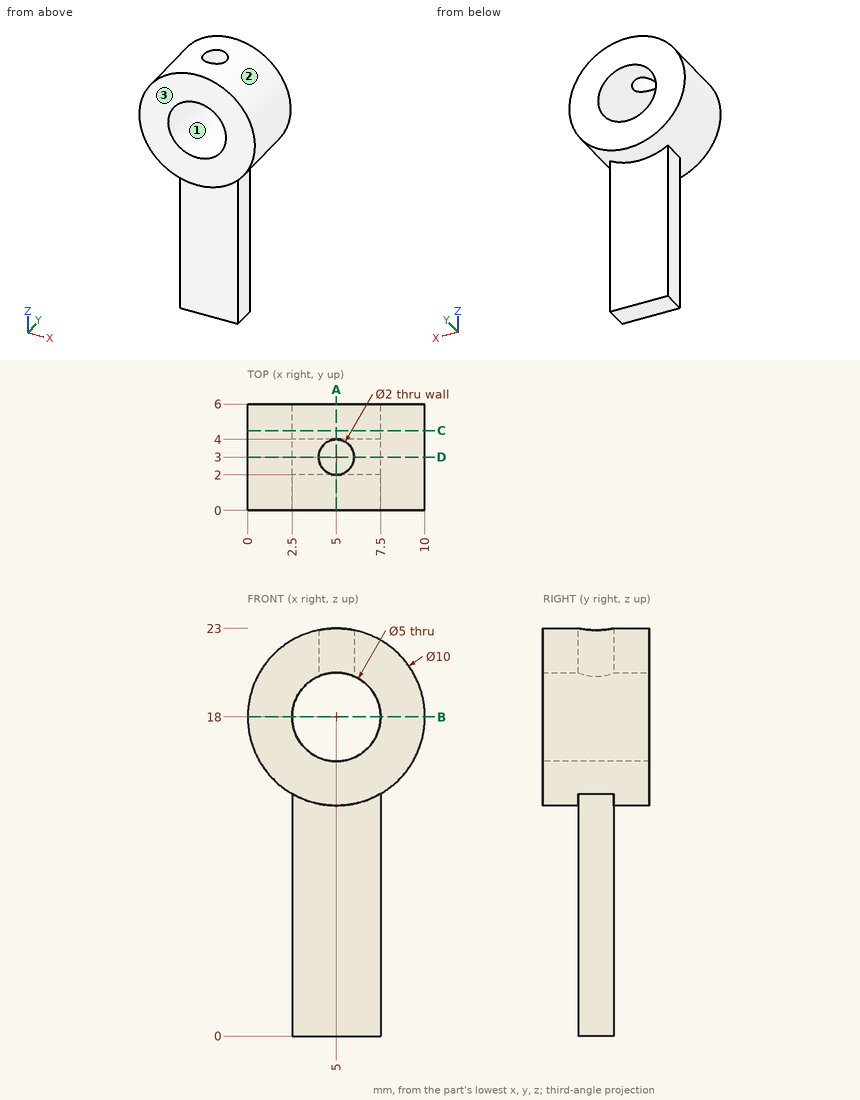
Design review of the part shown in the three views and the two pictorial views. Dimensions are in mm from the part's minimum x, y and z. Round coordinates to 2 decimals unless told otherwise and drop trailing zeros. Write each loop counter-clockwise with the first axis right and the second up, starting at its lowest first coordinate (ties: lowest second). Pieces come first, ordered by that corner, then holes. Notation, with made-up numbers: (-3, 27) -> (53, 27) arc R22 cw to (53, 46) -> close; hole circle Ø6 at (-21.75, 85). An arc over 180 degrees is marked (long way). Answer as a JSON object with one key per item and string values.
1. We need section B-B on z = 18. State the section outline as (x, y) points.
Results found:
{"outline": "(0, 0) -> (2.5, 0) -> (2.5, 6) -> (0, 6) -> close; (7.5, 0) -> (10, 0) -> (10, 6) -> (7.5, 6) -> close"}
2. The part is to be moulded in two halves that separate along X. For the marked faces 1, 2 and 3, say which applies: pulls with the +X half, pulls with the -X half, needs draft (parallel to the pull), parting line crosses it, or undercut.
Results found:
{"face 1": "undercut", "face 2": "parting line crosses it", "face 3": "needs draft"}
3. We need section A-A on x = 5. State the section outline as (y, z) points, and give its area (3 significant figures).
Results found:
{"outline": "(0, 13) -> (2, 13) -> (2, 0) -> (4, 0) -> (4, 13) -> (6, 13) -> (6, 15.5) -> (0, 15.5) -> close; (0, 20.5) -> (2, 20.5) -> (2, 23) -> (0, 23) -> close; (4, 20.5) -> (6, 20.5) -> (6, 23) -> (4, 23) -> close", "area": "51.0 mm^2"}
4. To check wall thickness, follow line 1 along X through (y, z) = (1.25, 18); line 2 along Y through (x, z) = (3, 12.75); line 3 along Z through (x, y) = (6.25, 5.5). State the ranges of each line that lie inside material, in increasing order.
Results found:
{"line 1": "x = 0 to 2.5, 7.5 to 10", "line 2": "y = 2 to 4", "line 3": "z = 13.16 to 15.83, 20.17 to 22.84"}
5. Clearance check with flat-ended pins moving along their axes: pin 1 (1.8 mm diameter, centred on x = 5, y = 3, fed in from +Z); pin 2 (5.5 mm diameter, centred on x = 4.5, z = 4, fed in from -Y); pin 3 (1 mm diameter, centred on y = 5, z = 10, fed in from -X) (3 decimals); pin 4 (0.6 mm diameter, centred on y = 3.5, z = 10, fed in from -X). State where each tip first meets the part, or that it passes through.
Results found:
{"pin 1": "stops at z = 15.67", "pin 2": "stops at y = 2", "pin 3": "passes through", "pin 4": "stops at x = 2.5"}
6. We need section D-D on y = 3. State the section outline as (x, z) points.
Results found:
{"outline": "(2.5, 0) -> (7.5, 0) -> (7.5, 13.67) arc R5 ccw to (6, 22.9) -> (6, 20.29) arc R2.5 cw (long way) to (4, 20.29) -> (4, 22.9) arc R5 ccw to (2.5, 13.67) -> close"}
7. We need section C-C on y = 4.5. State the section outline as (x, z) points.
Results found:
{"outline": "circle Ø10 at (5, 18); hole circle Ø5 at (5, 18)"}
